Work out the finished part from the listing and answer in its coordinate system (mm). A direction names the side the tool comes from. Coordinates: 2 decimals unless noted, no trailing zeros. Order: outer loops, then holes, each group sorted by start corner. A loop starts at its lowest first (then second) coordinate and runs counter-clockwise, first axis right, second up. Notation, with made-up numbers: (60.25, -30.75) -> (71.25, -30.75) arc R9 cw to (71.25, -21.75) -> close; hole circle Ø3 at (-38, 61). An arc over 180 degrees is marked (long way). Write item = value, one per line. Start each with the question number.
Q1. Which of the six approach directions +Z, -Z, +X, -X, +Y, -Y give full straight-line access (tool end or side, diameter ignored) to faces 1 (the cylindrical face through (14.95, 12.07, 4.93)), 2 (the flat face through (-3.9, 14, -5.2))?
Q2. Flat-ended cylindrical pins translate along their axes: pin 1 (5 mm diameter, centred on x = 0, z = 0, fed in from -Y); pin 2 (4 mm diameter, centred on x = -1, z = 2, fed in from +Y); pin 3 (2 mm diameter, centred on y = 14, z = -8.5, fed in from +X). Find the tip coordinate at first contact, or state that the pin passes through.
Q3. The part is cut by section B-B, the plane y = 9.5. Determine the outline of the cut face in (x, z), plus the area to 3 significant figures.
Q4. The part is cut by section C-C, the plane z = 0. Determine the outline of the cut face in (x, y), plus the area to 3 significant figures.
Q5. Straight lines are drawn through the part: L1, parallel to Z at x = 16.5, y = 11.5; L2, parallel to Z at x = 0, y = 10.15; L3, parallel to X at y = 9.9, z = 0. For each, find the intervals that lie inside material, in ascending order. Write a range as from..to.
Q6. The part is cut by section A-A, the plane x = -16.5. Determine the outline of the cut face in (y, z), plus the area to 3 significant figures.
Q7. The part is cut by section D-D, the plane z = -5. Determine the outline of the cut face in (x, y).
Q8. For a pull along X with two mould halves and no side action, classify faces 3 (the cylindrical face through (14.95, 12.07, -5.07)), 4 (the cylindrical face through (21.07, 14.54, 9.5)), 5 (the flat face through (0, 12, -11)), 6 (the cylindrical face through (-18.05, 12.07, 4.93)) as +X half, -X half, draft (parallel to the pull), parting line (faces both ways), or undercut.
```python
from build123d import *

# Parameters (mm, degrees)
CROQUIS1_R              = 10
CROQUIS1_R_2            = 3.5
EXTRUIR1_DEPTH          = 12
CROQUIS2_W              = 45
CROQUIS2_H              = 22
SALIENTE_EXTRUIR1_DEPTH = 5
REDONDEO1_R             = 5
REDONDEO2_R             = 5
REDONDEO3_R             = 5
REDONDEO4_R             = 5
CROQUIS3_R              = 4.1
CORTAR_EXTRUIR1_DEPTH   = 45
CROQUIS4_R              = 1.55
CORTAR_EXTRUIR2_DEPTH   = 45
CROQUIS7_W              = 22.113905464
CROQUIS7_H              = 24
CORTAR_EXTRUIR4_DEPTH   = 70
CROQUIS8_W              = 45
CROQUIS8_H              = 22
SALIENTE_EXTRUIR2_DEPTH = 5
REDONDEO5_R             = 5
REDONDEO6_R             = 5
REDONDEO7_R             = 5
REDONDEO8_R             = 5
CROQUIS9_R              = 1.55
CROQUIS9_R_2            = 4.1
CORTAR_EXTRUIR5_DEPTH   = 15
CORTAR_EXTRUIR7_DEPTH   = 6


with BuildPart() as part:
    # Croquis1 → Extruir1 (new body)
    with BuildSketch(Plane(origin=(0, 0, 0), x_dir=(1, 0, 0), z_dir=(0, 1, 0))):
        Circle(CROQUIS1_R)
        Circle(CROQUIS1_R_2, mode=Mode.SUBTRACT)
    extrude(amount=EXTRUIR1_DEPTH)

    # Croquis2 → Saliente-Extruir1 (add)
    with BuildSketch(Plane(origin=(0, 12, 0), x_dir=(1, 0, 0), z_dir=(0, 1, 0))):
        Rectangle(CROQUIS2_W, CROQUIS2_H)
    extrude(amount=SALIENTE_EXTRUIR1_DEPTH)

    # Redondeo1
    redondeo1_edges = [part.edges().sort_by_distance(p)[0] for p in [
        (22.5, 14.5, -11),
    ]]
    fillet(redondeo1_edges, radius=REDONDEO1_R)

    # Redondeo2
    redondeo2_edges = [part.edges().sort_by_distance(p)[0] for p in [
        (22.5, 14.5, 11),
    ]]
    fillet(redondeo2_edges, radius=REDONDEO2_R)

    # Redondeo3
    redondeo3_edges = [part.edges().sort_by_distance(p)[0] for p in [
        (-22.5, 14.5, 11),
    ]]
    fillet(redondeo3_edges, radius=REDONDEO3_R)

    # Redondeo4
    redondeo4_edges = [part.edges().sort_by_distance(p)[0] for p in [
        (-22.5, 14.5, -11),
    ]]
    fillet(redondeo4_edges, radius=REDONDEO4_R)

    # Croquis3 → Cortar-Extruir1 (cut)
    with BuildSketch(Plane.XZ):
        Circle(CROQUIS3_R)
    extrude(amount=-CORTAR_EXTRUIR1_DEPTH, mode=Mode.SUBTRACT)

    # Croquis4 → Cortar-Extruir2 (cut)
    with BuildSketch(Plane.XZ.offset(-12)):
        with Locations((-16.5, 5)):
            Circle(CROQUIS4_R)
        with Locations((-16.5, -5)):
            Circle(CROQUIS4_R)
        with Locations((16.5, 5)):
            Circle(CROQUIS4_R)
        with Locations((16.5, -5)):
            Circle(CROQUIS4_R)
    extrude(amount=-CORTAR_EXTRUIR2_DEPTH, mode=Mode.SUBTRACT)

    # Croquis7 → Cortar-Extruir4 (cut)
    with BuildSketch(Plane.XY.offset(11)):
        Rectangle(CROQUIS7_W, CROQUIS7_H)
    extrude(amount=-CORTAR_EXTRUIR4_DEPTH, mode=Mode.SUBTRACT)

    # Croquis8 → Saliente-Extruir2 (add)
    with BuildSketch(Plane.XZ.offset(-12)):
        Rectangle(CROQUIS8_W, CROQUIS8_H)
    extrude(amount=SALIENTE_EXTRUIR2_DEPTH)

    # Redondeo5
    redondeo5_edges = [part.edges().sort_by_distance(p)[0] for p in [
        (-22.5, 9.5, -11),
    ]]
    fillet(redondeo5_edges, radius=REDONDEO5_R)

    # Redondeo6
    redondeo6_edges = [part.edges().sort_by_distance(p)[0] for p in [
        (22.5, 9.5, -11),
    ]]
    fillet(redondeo6_edges, radius=REDONDEO6_R)

    # Redondeo7
    redondeo7_edges = [part.edges().sort_by_distance(p)[0] for p in [
        (22.5, 9.5, 11),
    ]]
    fillet(redondeo7_edges, radius=REDONDEO7_R)

    # Redondeo8
    redondeo8_edges = [part.edges().sort_by_distance(p)[0] for p in [
        (-22.5, 9.5, 11),
    ]]
    fillet(redondeo8_edges, radius=REDONDEO8_R)

    # Croquis9 → Cortar-Extruir5 (cut)
    with BuildSketch(Plane(origin=(0, 17, 0), x_dir=(1, 0, 0), z_dir=(0, 1, 0))):
        with Locations((-16.5, -5)):
            Circle(CROQUIS9_R)
        with Locations((-16.5, 5)):
            Circle(CROQUIS9_R)
        with Locations((16.5, -5)):
            Circle(CROQUIS9_R)
        with Locations((16.5, 5)):
            Circle(CROQUIS9_R)
        Circle(CROQUIS9_R_2)
    extrude(amount=-CORTAR_EXTRUIR5_DEPTH, mode=Mode.SUBTRACT)

    # Croquis10 → Cortar-Extruir7 (cut)
    with BuildSketch(Plane(origin=(0, 17, 0), x_dir=(1, 0, 0), z_dir=(0, 1, 0))):
        Polygon((6.941222487, -2.855304489), (5.943377466, 4.583622763), (-0.997845021, 7.438927251), (-6.941222487, 2.855304489), (-5.943377466, -4.583622763), (0.997845021, -7.438927251), align=None)
    extrude(amount=-CORTAR_EXTRUIR7_DEPTH, mode=Mode.SUBTRACT)


solid = part.part
```
Model answer:
q1.face_1 = +Y, -Y
q1.face_2 = +Y
q2.pin_1 = through
q2.pin_2 = 11
q2.pin_3 = 22.27
q3.outline = (-22.5, -6) arc R5 ccw to (-17.5, -11) -> (17.5, -11) arc R5 ccw to (22.5, -6) -> (22.5, 6) arc R5 ccw to (17.5, 11) -> (-17.5, 11) arc R5 ccw to (-22.5, 6) -> close; hole circle Ø3.1 at (-16.5, -5); hole circle Ø3.1 at (-16.5, 5); hole circle Ø8.2 at (0, 0); hole circle Ø3.1 at (16.5, -5); hole circle Ø3.1 at (16.5, 5)
q3.area = 886 mm2
q4.outline = (-22.5, 7) -> (-4.1, 7) -> (-4.1, 11) -> (-6.56, 11) -> (-6.56, 17) -> (-22.5, 17) -> close; (4.1, 7) -> (22.5, 7) -> (22.5, 17) -> (6.56, 17) -> (6.56, 11) -> (4.1, 11) -> close
q4.area = 339 mm2
q5.L1 = -11..-6.55, -3.45..3.45, 6.55..11
q5.L2 = -11..-4.1, 4.1..11
q5.L3 = -22.5..-4.1, 4.1..22.5
q6.outline = (7, -11) -> (17, -11) -> (17, -6.55) -> (7, -6.55) -> close; (7, -3.45) -> (17, -3.45) -> (17, 3.45) -> (7, 3.45) -> close; (7, 6.55) -> (17, 6.55) -> (17, 11) -> (7, 11) -> close
q6.area = 158 mm2
q7.outline = (-22.5, 7) -> (-18.05, 7) -> (-18.05, 17) -> (-22.5, 17) -> close; (-14.95, 7) -> (14.95, 7) -> (14.95, 17) -> (4.93, 17) -> (4.93, 11) -> (-4.16, 11) -> (-4.16, 17) -> (-14.95, 17) -> close; (18.05, 7) -> (22.5, 7) -> (22.5, 17) -> (18.05, 17) -> close
q8.face_3 = undercut
q8.face_4 = +X half
q8.face_5 = draft
q8.face_6 = undercut
